The model under review builds one solid part; all positions refer to its coordinate system, in mm. Face numbers are marked on the shaded views. A direction names the side the tool comes from. Round coordinates to 2 decimals unless told otherwise and drop trailing zeros. Order: outer loops, then holes, each group sorted by start corner. A loop starts at its lowest first (then second) coordinate and runs counter-clockwise, first axis right, second up. Notation, with made-up numbers: M 35.5,9.25 L 39.5,9.25 A35 ccw 39.5,46.25 Z; hole C -22,-5.5 d11. An arc over 180 degrees is marked long. Answer as a JSON object with one key per item and string values. Group by question number.
1. Add section C-C on z = 96. State the section outline as (x, y) points, and give its area (3 significant figures).
2. Clearance check with flat-ended pins moving along their axes: P1, Ø4, axis at x = -33, z = 35.5, coming from the -Y side; P2, Ø6, axis at x = 67, z = 71, coming from the +Y side; P3, Ø9.5, axis at y = 23.5, z = 89.5, coming from the +X side. State where each tip first meets the part, or that it passes through.
3. Machinability: for the marked faces 1, 2, 3, 4 and 5, which of the approach directions +Z, -Z, +X, -X, +Y, -Y give a long, thin tool a straight path to every point of the face, cutting with its end or side? Answer none if there is none.
4. Add section A-A on x = -9. State the section outline as (y, z) points.
5. Add section D-D on x = -47. State the section outline as (y, z) points, and give its area (3 significant figures).
6. Add section B-B on y = 13. State the section outline as (x, z) points.
7. To check wall thickness, follow probe 1 along Z at (x, y) = (36.5, 24.5); probe 2 along Z at (x, y) = (-0.5, 27.5); probe 3 along X at (y, z) = (12.5, 98.5). State the ranges of each line that lie inside material, in increasing order. Write a range as [from, to].
```python
from build123d import *

# Parameters (mm, degrees)
BOSS_EXTRUDE1_DEPTH = 180
CUT_EXTRUDE1_DEPTH  = 207.548420473
BOSS_EXTRUDE2_DEPTH = 175
CUT_EXTRUDE5_DEPTH  = 180
CUT_EXTRUDE6_DEPTH  = 180
SKETCH7_W           = 55
SKETCH7_H           = 24
CUT_EXTRUDE7_DEPTH  = 180
SKETCH8_W           = 55
SKETCH8_H           = 50
CUT_EXTRUDE8_DEPTH  = 180
FILLET1_R           = 12
FILLET2_R           = 12
FILLET3_R           = 12
FILLET4_R           = 12
FILLET5_R           = 5
FILLET6_R           = 5
FILLET7_R           = 5
FILLET8_R           = 5


with BuildPart() as part:
    # Sketch1 → Boss-Extrude1 (new body)
    with BuildSketch(Plane.XY):
        Polygon((-75.25, 0), (75.25, 0), (75.25, 16), (90, 46.5), (-90, 46.5), (-75.25, 16), align=None)
    extrude(amount=BOSS_EXTRUDE1_DEPTH)

    # Sketch2 → Cut-Extrude1 (cut, through all)
    with BuildSketch(Plane.XY.offset(180)):
        Polygon((-51.25, 0), (-60.372134253, 15.8), (-50.372134253, 15.8), (-50.372134253, 17.3), (49.372134253, 17.3), (49.372134253, 15.8), (64.372134253, 15.8), (55.25, 0), align=None)
    extrude(amount=-CUT_EXTRUDE1_DEPTH, mode=Mode.SUBTRACT)


with BuildPart() as body_2:
    # Sketch3 → Boss-Extrude2 (new body)
    with BuildSketch(Plane.XY.offset(180)):
        Polygon((90, 46.5), (75.25, 16), (90, 16), align=None)
    extrude(amount=-BOSS_EXTRUDE2_DEPTH)


with BuildPart() as cut_extrude5_tool:
    # Sketch5 → Cut-Extrude5 (new body)
    with BuildSketch(Plane(origin=(90, 0, 0), x_dir=(0, 0, -1), z_dir=(1, 0, 0))):
        Polygon((-156, 46.5), (-165.237604307, 30.5), (-150.237604307, 30.5), (-150.237604307, 29), (-25.18556724, 29.732954619), (-25.18556724, 31.232954619), (-15.18556724, 31.232954619), (-24, 46.5), align=None)
    extrude(amount=-CUT_EXTRUDE5_DEPTH)


with BuildPart() as part_1:
    add(part.part)

    # Cut-Extrude5: cut by cut_extrude5_tool
    add(cut_extrude5_tool.part, mode=Mode.SUBTRACT)

    # Sketch7 → Cut-Extrude7 (cut)
    with BuildSketch(Plane(origin=(0, 29.879545719, 0.175129902), x_dir=(1, 0, 0), z_dir=(0, 0.9999828236276607, 0.005861096284045548))):
        with Locations((0, -47.727459023)):
            Rectangle(SKETCH7_W, SKETCH7_H)
    extrude(amount=-CUT_EXTRUDE7_DEPTH, mode=Mode.SUBTRACT)

    # Sketch8 → Cut-Extrude8 (cut)
    with BuildSketch(Plane(origin=(0, 29.879545719, 0.175129902), x_dir=(1, 0, 0), z_dir=(0, 0.9999828236276607, 0.005861096284045548))):
        with Locations((30.72704543, -89.724367276)):
            Rectangle(SKETCH8_W, SKETCH8_H)
    extrude(amount=-CUT_EXTRUDE8_DEPTH, mode=Mode.SUBTRACT)

    # Fillet1
    fillet1_edges = [part_1.edges().sort_by_distance(p)[0] for p in [
        (-27.5, 23.414738665, 59.865723337),
    ]]
    fillet(fillet1_edges, radius=FILLET1_R)

    # Fillet2
    fillet2_edges = [part_1.edges().sort_by_distance(p)[0] for p in [
        (-27.5, 23.485071821, 35.865723333),
    ]]
    fillet(fillet2_edges, radius=FILLET2_R - 0.0001)  # a hair under: the kernel refuses the full size

    # Fillet3
    fillet3_edges = [part_1.edges().sort_by_distance(p)[0] for p in [
        (27.5, 23.414738665, 59.865723337),
    ]]
    fillet(fillet3_edges, radius=FILLET3_R)

    # Fillet4
    fillet4_edges = [part_1.edges().sort_by_distance(p)[0] for p in [
        (27.5, 23.485071821, 35.865723333),
    ]]
    fillet(fillet4_edges, radius=FILLET4_R - 0.0001)  # a hair under: the kernel refuses the full size

    # Fillet5
    fillet5_edges = [part_1.edges().sort_by_distance(p)[0] for p in [
        (58.22704543, 22.650094985, 64.858235693),
    ]]
    fillet(fillet5_edges, radius=FILLET5_R)

    # Fillet6
    fillet6_edges = [part_1.edges().sort_by_distance(p)[0] for p in [
        (3.22704543, 23.400094985, 64.86263159),
    ]]
    fillet(fillet6_edges, radius=FILLET6_R)

    # Fillet7
    fillet7_edges = [part_1.edges().sort_by_distance(p)[0] for p in [
        (3.22704543, 23.253567578, 114.862631598),
    ]]
    fillet(fillet7_edges, radius=FILLET7_R)

    # Fillet8
    fillet8_edges = [part_1.edges().sort_by_distance(p)[0] for p in [
        (58.22704543, 22.503567578, 114.8582357),
    ]]
    fillet(fillet8_edges, radius=FILLET8_R)


with BuildPart() as body_2_1:
    add(body_2.part)

    # Cut-Extrude5: cut by cut_extrude5_tool
    add(cut_extrude5_tool.part, mode=Mode.SUBTRACT)

    # Sketch6 → Cut-Extrude6 (cut)
    with BuildSketch(Plane.XY.offset(180)):
        Polygon((75.25, 16), (90, 46.5), (90, 16), align=None)
    extrude(amount=-CUT_EXTRUDE6_DEPTH, mode=Mode.SUBTRACT)


solid = part_1.part
```
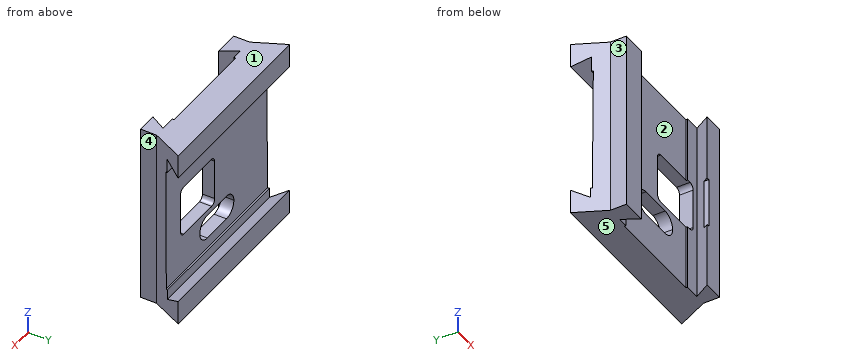
Recorded:
{
 "1": {"outline": "M -81.69,29.32 L -75.25,16 L -75.25,0 L -51.25,0 L -60.37,15.8 L -50.37,15.8 L -50.37,17.3 L 3.23,17.3 L 3.23,29.32 Z; M 58.23,0 L 75.25,0 L 75.25,16 L 81.69,29.32 L 58.23,29.32 L 58.23,15.8 L 64.37,15.8 L 58.23,5.16 Z", "area": "1,840 mm²"},
 "2": {"P1": "stops at y = 17.3", "P2": "stops at y = 29.48", "P3": "stops at x = 81.17"},
 "3": {"face 1": "+Z, +X, -X, +Y, -Y", "face 2": "+Z, -Z, -Y", "face 3": "+Z, -Z, -X, -Y", "face 4": "+Z, -Z, +X, -Y", "face 5": "-Z, +X, -X, +Y, -Y"},
 "4": {"outline": "M 17.3,0 L 46.5,0 L 46.5,24 L 31.23,15.19 L 31.23,25.19 L 29.73,25.19 L 29.67,35.9 L 17.3,35.83 Z; M 17.3,59.83 L 29.53,59.9 L 29,150.24 L 30.5,150.24 L 30.5,165.24 L 46.5,156 L 46.5,180 L 17.3,180 Z"},
 "5": {"outline": "M 17.3,0 L 46.5,0 L 46.5,24 L 31.23,15.19 L 31.23,25.19 L 29.73,25.19 L 29,150.24 L 30.5,150.24 L 30.5,165.24 L 46.5,156 L 46.5,180 L 17.3,180 Z", "area": "2,860 mm²"},
 "6": {"outline": "M -75.25,0 L -58.76,0 L -58.76,180 L -75.25,180 Z; M 62.76,0 L 75.25,0 L 75.25,180 L 62.76,180 Z"},
 "7": {"probe 1": "z = [0, 64.87], [114.87, 180]", "probe 2": "z = [0, 35.89], [59.89, 180]", "probe 3": "x = [-75.25, -58.47], [62.47, 75.25]"}
}
